The listing builds one solid part. Answer for the finished solid, in the listing's coordinates (mm). Face numbers are marked on the shaded views. A direction names the side the tool comes from. Round coordinates to 2 decimals unless told otherwise and drop trailing zeros. Loops run counter-clockwise (first coordinate to the right, second up) from the corner with the lowest first, then second, coordinate; pieces in that order, holes last. Notation, with made-up numbers: (49.25, 59.25) -> (68.25, 59.25) arc R22 cw to (68.25, 84.25) -> close; hole circle Ø5 at (-5.75, -8.75). An arc over 180 degrees is marked (long way). Write each question's results on one line, items separated by ' | '. Start each with the question number.
(1) The part is cut by section C-C (z = 3.9). Determine the outline of the cut face in (x, y), plus the area to 3 significant figures.
(2) The part is cut by section A-A (z = 0.6). Determine the outline of the cut face in (x, y), plus the area to 3 significant figures.
(3) The part is cut by section B-B (x = 0). Determine the outline of the cut face in (y, z).
(4) The part is cut by section D-D (y = -3.25). Determine the outline of the cut face in (x, z).
(5) Determine the mould class of the marked faces 4, 5, 6 and 7 for opening direction X: released by +X, released by -X, zero draft, split by the parting line, or undercut.
(6) Straight lines are drawn through the part: probe 1 along Y at (x, z) = (0, 1.05); probe 2 along X at (y, z) = (0, 2.9); probe 3 along Y at (x, z) = (12, 2.8). For each, find the intervals that lie inside material, in ascending order.
(7) Flat-ended cylindrical pins translate along their axes: pin 1 (1.2 mm diameter, centred on x = 12, y = 0, fed in from -Z); pin 2 (2 mm diameter, centred on x = 0, y = 0, fed in from +Z); pin 3 (0.9 mm diameter, centred on x = -8, y = 0, fed in from -Z). Find the tip coordinate at first contact, or state that the pin passes through.
(8) For the marked faces 1, 2 and 3, determine the directions among +Z, -Z, +X, -X, +Y, -Y from which every point of the face is accessible in a straight line to the end or side of a thin tool.
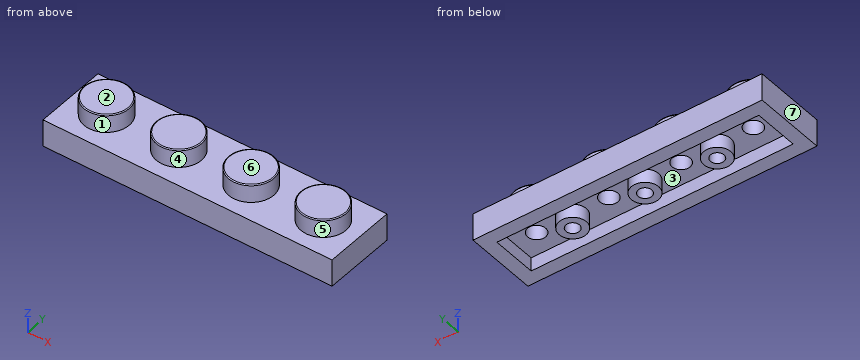
```python
from build123d import *

# Parameters (mm, degrees)
F0_W     = 32
F0_H     = 8
F1_DEPTH = 3
F2_R     = 2.5
F3_DEPTH = 2
F4_R     = 0.1
F5_T     = -1.5
F6_R     = 1.5
F6_R_2   = 0.75
F7_DEPTH = 1.5


# Not quite as in the source:
# - a feature names something its author has since deleted; it is built from what else it names


with BuildPart() as f1:
    # F0 (on Top) → F1 (new body)
    with BuildSketch(Plane.XY):
        Rectangle(F0_W, F0_H)
    extrude(amount=F1_DEPTH)

    # F2 (on face) → F3 (join)
    with BuildSketch(Plane.XY.offset(3)):
        with Locations((-12, 0)):
            Circle(F2_R)
        with Locations((-4, 0)):
            Circle(F2_R)
        with Locations((4, 0)):
            Circle(F2_R)
        with Locations((12, 0)):
            Circle(F2_R)
    extrude(amount=F3_DEPTH)

    # F4
    f4_edges = [f1.edges().sort_by_distance(p)[0] for p in [
        (-14.5, 0, 5),
        (-6.5, 0, 5),
        (1.5, 0, 5),
        (9.5, 0, 5),
    ]]
    fillet(f4_edges, radius=F4_R)

    # F5
    f5_openings = [f1.faces().sort_by_distance(p)[0] for p in [
        (0, 0, 0),
    ]]
    offset(amount=F5_T, openings=f5_openings, kind=Kind.INTERSECTION)

    # F6 (on face) → F7 (join, through all)
    with BuildSketch(Plane(origin=(0, 0, 1.5), x_dir=(1, 0, 0), z_dir=(0, 0, -1))):
        with Locations((-8, 0)):
            Circle(F6_R)
        with Locations((-8, 0)):
            Circle(F6_R_2, mode=Mode.SUBTRACT)
        Circle(F6_R)
        Circle(F6_R_2, mode=Mode.SUBTRACT)
        with Locations((8, 0)):
            Circle(F6_R)
        with Locations((8, 0)):
            Circle(F6_R_2, mode=Mode.SUBTRACT)
    extrude(amount=F7_DEPTH)


solid = f1.part
```
Checked values:
1) outline: circle Ø5 at (-12, 0); circle Ø5 at (-4, 0); circle Ø5 at (4, 0); circle Ø5 at (12, 0) | area: 78.5 mm2
2) outline: (-16, -4) -> (16, -4) -> (16, 4) -> (-16, 4) -> close; circle Ø3 at (-8, 0); circle Ø3 at (0, 0); circle Ø3 at (8, 0); hole (-14.5, -2.5) -> (14.5, -2.5) -> (14.5, 2.5) -> (-14.5, 2.5) -> close; hole circle Ø1.5 at (-8, 0); hole circle Ø1.5 at (0, 0); hole circle Ø1.5 at (8, 0) | area: 127 mm2
3) outline: (-4, 0) -> (-2.5, 0) -> (-2.5, 1.5) -> (-1.5, 1.5) -> (-1.5, 0) -> (-0.75, 0) -> (-0.75, 1.5) -> (0.75, 1.5) -> (0.75, 0) -> (1.5, 0) -> (1.5, 1.5) -> (2.5, 1.5) -> (2.5, 0) -> (4, 0) -> (4, 3) -> (-4, 3) -> close
4) outline: (-16, 0) -> (16, 0) -> (16, 3) -> (-16, 3) -> close
5) face 4: undercut | face 5: undercut | face 6: zero draft | face 7: released by -X
6) probe 1: y = -4 to -2.5, -1.5 to -0.75, 0.75 to 1.5, 2.5 to 4 | probe 2: x = -16 to -13, -11 to -5, -3 to 3, 5 to 11, 13 to 16 | probe 3: y = -4 to -1, 1 to 4
7) pin 1: stops at z = 3.5 | pin 2: stops at z = 3 | pin 3: stops at z = 1.5
8) face 1: +Z | face 2: +Z, +X, -X, +Y, -Y | face 3: -Z
